Autodesk Inventor part; units mm, degrees
ref_plane "YZ Plane" through (0, 0, 0) normal (1, 0, 0) x (0, 1, 0)
ref_plane "XZ Plane" through (0, 0, 0) normal (0, 1, 0) x (-1, 0, 0)
ref_plane "XY Plane" through (0, 0, 0) normal (0, 0, 1) x (1, 0, 0)
sketch "Sketch1" plane through (0, 0, 0) normal (1, 0, 0) x (0, 1, 0)
  line L0 (0, 0) -> (65, 0)
  line L1 (65, -35) -> (0, -35)
  line L2 (65, -14) -> (71, -14)
  line L3 (71, -14) -> (71, -21)
  line L4 (71, -21) -> (65, -21)
  line L5 (0, -14) -> (-6, -14)
  line L6 (-6, -14) -> (-6, -21)
  line L7 (-6, -21) -> (0, -21)
  line L8 (65, 0) -> (65, -14)
  line L9 (65, -21) -> (65, -35)
  line L10 (0, -35) -> (0, -21)
  line L11 (0, -14) -> (0, 0)
  line L12 (32.5, -17.5) -> (22.5, -17.5)
  circle A0 centre (42.5, -17.5) radius 2.1
  circle A1 centre (22.5, -17.5) radius 2.1
  dimension "d0" = 65
  dimension "d1" = 35
  dimension "d3" = 6
  dimension "d4" = 7
  dimension "d6" = 6
  dimension "d7" = 7
  dimension "d8" = 10
  dimension "d10" = 4.2
  dimension "d11" = 4.2
extrude "Extrusion1" add sketch "Sketch1" along normal blind 6
sketch "Sketch2" plane through (6, 0, 0) normal (1, 0, 0) x (0, 0, -1)
  line L0 (14, 65) -> (0, 65)
  line L1 (0, 65) -> (0, 58.5)
  line L2 (0, 65) -> (0, 0)
  line L3 (0, 58.5) -> (6, 58.5)
  line L4 (6, 58.5) -> (6, 52)
  line L5 (6, 52) -> (0, 52)
  line L6 (0, 52) -> (0, 58.5)
  line L7 (35, 65) -> (35, 58.5)
  line L8 (35, 0) -> (35, 65)
  line L9 (35, 58.5) -> (29, 58.5)
  line L10 (29, 58.5) -> (29, 52)
  line L11 (29, 52) -> (35, 52)
  line L12 (35, 52) -> (35, 58.5)
  dimension "d15" = 6.5
  dimension "d16" = 6
  dimension "d17" = 6.5
  dimension "d18" = 6.5
  dimension "d19" = 6
  dimension "d20" = 6.5
extrude "Extrusion2" cut sketch "Sketch2" against normal blind 10
pattern_linear "Rectangular Pattern1" count 5 spacing 13 along (0, -1, 0) of "Extrusion2"
sketch "Sketch3" plane through (6, 0, 0) normal (1, 0, 0) x (0, 0, -1)
  circle A0 centre (17.5, 42.5) radius 2.1
  circle A1 centre (17.5, 32.5) radius 5
  point P0 (0, 0)
  dimension "d27" = 10
extrude "Extrusion3" cut sketch "Sketch3" against normal blind 10 contours A1
properties part number "g_arm_v_2"
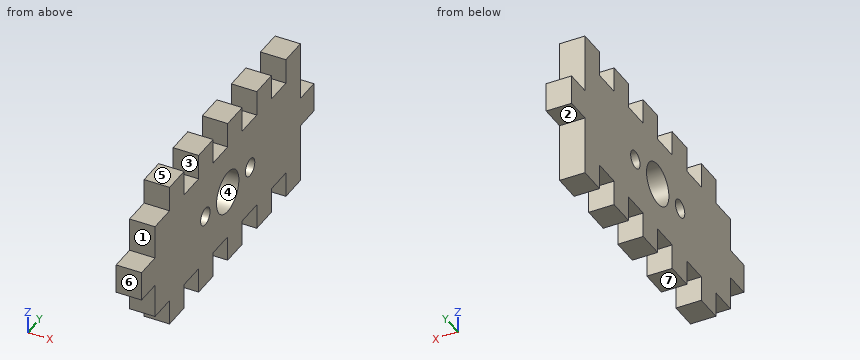
Input: part model. Units: mm. Frame: model coordinates. Face numbers are marked on the shaded views. A direction names the side the tool comes from. Round coordinates to 2 decimals unless told otherwise and drop trailing zeros. Write each loop counter-clockwise with the first axis right and the second up, starting at its lowest first coordinate (ties: lowest second). Pieces come first, ordered by that corner, then holes.
1) Contact query for flat-ended pins moving along their axis: P1, Ø3, axis at x = 2.5, z = -3.5, coming from the +Y side; P2, Ø1.8, axis at x = 2.5, y = 55.5, coming from the +Z side; P3, Ø8, axis at y = 32.5, z = -17.5, coming from the +X side. Output: stop coordinate, or through.
2) Draft query along Z for the marked faces 4, 5, 6 and 7. Return one class per face: pulls with the +Z half, pulls with the -Z half, needs draft (parallel to the pull), parting line crosses it, or undercut.
3) Cut plane A-A (z = -17.5). Return the cut outline in (x, y).
4) Cut plane C-C (z = -32). Return the cut outline in (x, y), then the cut area to 3 significant figures.
5) Cut plane B-B (y = 22.5). Return the cut outline in (x, z), then the cut area to 3 significant figures.
6) Cut plane D-D (x = 1.65). Count the separate pieces of the cut face and the enclosed holes in it, then the cut area to 3 significant figures.
7) Reachability of the marked faces 1, 2 and 3 from +Z, -Z, +X, -X, +Y, -Y: full face, straight path, thin tool, end or side. Return the list, or none.
8) Ray query, L1, parallel to Y at x = 1.2, z = -32; L2, parallel to Z at x = 1.3, y = 22.5; L3, parallel to Z at x = 2.25, y = 43.5. Return the intervals inside material, ascending.
Geometry says:
1. P1: stops at y = 65
1. P2: stops at z = -6
1. P3: passes through
2. face 4: undercut
2. face 5: pulls with the +Z half
2. face 6: needs draft
2. face 7: pulls with the -Z half
3. outline: (0, -6) - (6, -6) - (6, 20.4) - (0, 20.4) - close; (0, 24.6) - (6, 24.6) - (6, 27.5) - (0, 27.5) - close; (0, 37.5) - (6, 37.5) - (6, 40.4) - (0, 40.4) - close; (0, 44.6) - (6, 44.6) - (6, 71) - (0, 71) - close
4. outline: (0, 6.5) - (6, 6.5) - (6, 13) - (0, 13) - close; (0, 19.5) - (6, 19.5) - (6, 26) - (0, 26) - close; (0, 32.5) - (6, 32.5) - (6, 39) - (0, 39) - close; (0, 45.5) - (6, 45.5) - (6, 52) - (0, 52) - close; (0, 58.5) - (6, 58.5) - (6, 65) - (0, 65) - close
4. area: 195 mm2
5. outline: (0, -35) - (6, -35) - (6, -19.6) - (0, -19.6) - close; (0, -15.4) - (6, -15.4) - (6, 0) - (0, 0) - close
5. area: 185 mm2
6. separate pieces: 1
6. enclosed holes: 3
6. area: 1,860 mm2
7. face 1: +Z, +X, -X, -Y
7. face 2: -Z, +X, -X, +Y
7. face 3: +Z, +X, -X
8. L1: y = 6.5 to 13, 19.5 to 26, 32.5 to 39, 45.5 to 52, 58.5 to 65
8. L2: z = -35 to -19.6, -15.4 to 0
8. L3: z = -29 to -19.35, -15.65 to -6
